```python
from build123d import *

# Parameters (mm, degrees)
F2_W     = 10
F2_H     = 4
F2_R     = 1.4
F3_DEPTH = 5
F4_W     = 10
F4_H     = 4
F4_R     = 1.4
F5_DEPTH = 5


with BuildPart() as f1:
    # F0 (on Front) → F1 (revolve)
    with BuildSketch(Plane.XZ):
        with BuildLine():
            Line((1.4, 7.5), (0, 7.5))
            Line((0, 7.5), (0, 0))
            Line((0, 0), (0, -7.5))
            Line((0, -7.5), (1.4, -7.5))
            Line((1.4, -7.5), (1.4, -0.4))
            Line((1.4, -0.4), (1.15, -0.4))
            ThreePointArc((1.15, -0.4), (0.8671572875, -0.2828427125), (0.75, 0))
            ThreePointArc((0.75, 0), (0.8671572875, 0.2828427125), (1.15, 0.4))
            Line((1.15, 0.4), (1.4, 0.4))
            Line((1.4, 0.4), (1.4, 7.5))
        make_face()
    revolve(axis=Axis((0, 0, 3.75), (0, 0, 1)))

    # F2 (on face) → F3 (join)
    with BuildSketch(Plane.XY.offset(7.5)):
        Rectangle(F2_W, F2_H)
        Circle(F2_R, mode=Mode.SUBTRACT)
        Circle(F2_R)
    extrude(amount=F3_DEPTH)

    # F4 (on face) → F5 (join)
    with BuildSketch(Plane(origin=(0, 0, -7.5), x_dir=(1, 0, 0), z_dir=(0, 0, -1))):
        Rectangle(F4_W, F4_H)
        Circle(F4_R, mode=Mode.SUBTRACT)
        Circle(F4_R)
    extrude(amount=F5_DEPTH)


solid = f1.part
```
Geometry check sheet. Reference: the model listing, model coordinates, mm. A direction names the side the tool comes from. Give positions to 0.01 mm unless a question says otherwise; leave off trailing zeros. Order: outer loops, then holes, each group sorted by start corner. A loop starts at its lowest first (then second) coordinate and runs counter-clockwise, first axis right, second up. Notation, with made-up numbers: (-15.75, 18) - (21.25, 18) arc R27 ccw to (21.25, 51) - close; hole circle Ø5 at (-2, -31.75). An arc over 180 degrees is marked (long way). Write item = value, one per line. Start each with the question number.
1) Gauge pin test, flat ends, axial feed: pin 1 Ø2 at (y, z) = (-1, 2.5) entering from +X; pin 2 Ø5 at (x, z) = (-1, 5.5) entering from -Y. Record the tip position at first contact, or that the pin passes through.
2) Access from +Z, -Z, +X, -X, +Y, -Y to the whole of each face (thin tool, end or side, straight path). Record for faces 5 (the flat face through (-5, 0, -10)), 6 (the cylindrical face through (-1.4, 0.06, -3.9)).
3) Draft check along Z on faces 1 (the flat face through (0, 0, -12.5)), 2 (the flat face through (0, -2, -10)), 3 (the flat face through (0, 0, 12.5)), 4 (the flat face through (-1.2, 1.4, 7.5)). Enter one of: released by +Z, released by -Z, zero draft, split by the parting line, or undercut.
4) Section check A-A (x = -4.25). Enter the section's corners in (y, z), then the cut area to 3 significant figures.
5) Section check B-B (z = 6). Enter the section's corners in (x, y).
6) Scan lines: L1, parallel to Z at x = 0.5, y = 1.5; L2, parallel to X at y = -0.1, z = 5.25; L3, parallel to Y at x = 0.5, z = 2. Record each from-to range of solid material in increasing order.
Geometry check:
q1.pin_1 = 1.4
q1.pin_2 = -2
q2.face_5 = +Z, -Z, -X, +Y, -Y
q2.face_6 = none
q3.face_1 = released by -Z
q3.face_2 = zero draft
q3.face_3 = released by +Z
q3.face_4 = undercut
q4.outline = (-2, -12.5) - (2, -12.5) - (2, -7.5) - (-2, -7.5) - close; (-2, 7.5) - (2, 7.5) - (2, 12.5) - (-2, 12.5) - close
q4.area = 40.0 mm2
q5.outline = circle Ø2.8 at (0, 0)
q6.L1 = -12.5 to -7.5, 7.5 to 12.5
q6.L2 = -1.4 to 1.4
q6.L3 = -1.31 to 1.31
